Verification items for the finished model (mm, model axes). A direction names the side the tool comes from. Coordinates: 2 decimals unless noted, no trailing zeros. Order: outer loops, then holes, each group sorted by start corner. A loop starts at its lowest first (then second) coordinate and runs counter-clockwise, first axis right, second up. Notation, with made-up numbers: (61, 73.25) -> (109, 73.25) arc R11 ccw to (109, 80.25) -> close; hole circle Ø4 at (-33.75, -12). An arc over 180 degrees is marked (long way). Answer as CSV lines item,"result".
```python
from build123d import *

# Parameters (mm, degrees)
BOSS_EXTRUDE1_START = -2.1
SKETCH1_R           = 3
BOSS_EXTRUDE1_DEPTH = 2
CUT_EXTRUDE1_DEPTH  = 3
SKETCH3_R           = 0.5
CUT_EXTRUDE2_DEPTH  = 3


with BuildPart() as part:
    # Sketch1 → Boss-Extrude1 (new body)
    with BuildSketch(Plane.XY.offset(BOSS_EXTRUDE1_START)):
        Circle(SKETCH1_R)
    extrude(amount=BOSS_EXTRUDE1_DEPTH)

    # Sketch2 → Cut-Extrude1 (cut, through all)
    with BuildSketch(Plane.XY.offset(-0.1)):
        with BuildLine():
            Line((0.25, 1.224744871), (0.25, 2.210910446))
            ThreePointArc((0.25, 2.210910446), (-2.225, 0), (0.25, -2.210910446))
            Line((0.25, -2.210910446), (0.25, -1.224744871))
            ThreePointArc((0.25, -1.224744871), (1.25, 0), (0.25, 1.224744871))
        make_face()
    extrude(amount=-CUT_EXTRUDE1_DEPTH, mode=Mode.SUBTRACT)

    # Sketch3 → Cut-Extrude2 (cut, through all)
    with BuildSketch(Plane.XY.offset(-0.1)):
        with Locations((1.414213562, 1.414213562)):
            Circle(SKETCH3_R)
    cut_extrude2 = extrude(amount=-CUT_EXTRUDE2_DEPTH, mode=Mode.SUBTRACT)

    # Mirror1: Cut-Extrude2 across plane
    add(cut_extrude2.mirror(Plane.ZX), mode=Mode.SUBTRACT)


solid = part.part
```
Item 1: Release check for a two-part mould opening along X. For faces 1 (the flat face through (1.3, -0.6, -2.1)), 2 (the cylindrical face through (-3, 0, -1)), 3 (the cylindrical face through (1.25, -0.02, -1.09)) record: +X half, -X half, draft (parallel to the pull), parting line (faces both ways), or undercut.
Answer list:
face 1,"draft"
face 2,"parting line"
face 3,"undercut"
Item 2: Tool access check on faces 4 (the flat face through (1.3, -0.6, -0.1)), 5 (the flat face through (0.25, -2, -1)). Record the directions out of +Z, -Z, +X, -X, +Y, -Y that give a thin tool (end or side, any length) a straight path to the whole face; none if there is none.
Answer list:
face 4,"+Z, +X, -X, +Y, -Y"
face 5,"+Z, -Z"
Item 3: Section check C-C, the plane z = -1.5. Record the boundary of the cut face in (x, y) (3 decimals), plus the area to 3 significant figures.
Answer list:
outline,"circle Ø6 at (0, 0); hole (0.25, -2.211) -> (0.25, -1.225) arc R1.25 ccw to (0.25, 1.225) -> (0.25, 2.211) arc R2.225 ccw (long way) to start; hole circle Ø1 at (1.414, -1.414); hole circle Ø1 at (1.414, 1.414)"
area,"16.0 mm2"
Item 4: Section check D-D, the plane y = -1.15. Record the boundary of the cut face in (x, z).
Answer list:
outline,"(-2.77, -2.1) -> (-1.9, -2.1) -> (-1.9, -0.1) -> (-2.77, -0.1) -> close; (0.49, -2.1) -> (0.99, -2.1) -> (0.99, -0.1) -> (0.49, -0.1) -> close; (1.84, -2.1) -> (2.77, -2.1) -> (2.77, -0.1) -> (1.84, -0.1) -> close"
Item 5: Depth check by flat-ended pin: pin 1 Ø1 at (y, z) = (-1.5, -1.5) entering from +X; pin 2 Ø1 at (x, y) = (-0.5, -0.5) entering from -Z; pin 3 Ø1.1 at (y, z) = (-1.5, -1.5) entering from -X; pin 4 Ø0.8 at (y, z) = (2, -1.5) entering from -X. Enter the tip coordinate at first touch or a pass-through.
Answer list:
pin 1,"x = 2.83"
pin 2,"through"
pin 3,"x = -2.85"
pin 4,"x = -2.54"
Item 6: Thickness scan on line 1 (Y direction, x = 0, z = -1.3) (3 decimals); line 2 (Y direction, x = 1.3, z = -0.75); line 3 (Y direction, x = 1.6, z = -1.9). Record the ranges inside material, lowest first.
Answer list:
line 1,"-3 to -2.225, 2.225 to 3"
line 2,"-2.7 to -1.9, -0.93 to 0.93, 1.9 to 2.7"
line 3,"-2.54 to -1.88, -0.95 to 0.95, 1.88 to 2.54"
Item 7: Section check B-B, the plane x = 0. Record the boundary of the cut face in (y, z) (3 decimals), plus the area to 3 significant figures.
Answer list:
outline,"(-3, -2.1) -> (-2.225, -2.1) -> (-2.225, -0.1) -> (-3, -0.1) -> close; (2.225, -2.1) -> (3, -2.1) -> (3, -0.1) -> (2.225, -0.1) -> close"
area,"3.10 mm2"
Item 8: Section check A-A, the plane y = 0. Record the boundary of the cut face in (x, z) (3 decimals).
Answer list:
outline,"(-3, -2.1) -> (-2.225, -2.1) -> (-2.225, -0.1) -> (-3, -0.1) -> close; (1.25, -2.1) -> (3, -2.1) -> (3, -0.1) -> (1.25, -0.1) -> close"
